Verification items for this drawing (mm, ordinates from the low corner). A direction names the side the tool comes from. Coordinates: 2 decimals unless noted, no trailing zeros. Order: outer loops, then holes, each group sorted by start corner. A loop starts at its lowest first (then second) coordinate and runs counter-clockwise, first axis right, second up. Notation, with made-up numbers: M 63.5,-25 L 81.5,-25 A26 ccw 81.5,0 Z; hole C -16.75,74 d4. An arc over 180 degrees is marked long. Answer as a JSON object with one key per item and string values. Group by question number.
(1) Cross-section at A-A (y = 108). Enter the section's corners in (x, z).
(2) Gauge pin test, flat ends, axial feed: pin 1 Ø5 at (x, y) = (250.83, 7.17) entering from -Z; pin 2 Ø7 at (x, y) = (250.83, 140.83) entering from +Z. Record the tip position at first contact, or that the pin passes through.
(3) Cross-section at B-B (x = 163). Enter the section's corners in (y, z).
(4) Cross-section at C-C (z = 27.5). Enter the section's corners in (x, y), plus the area to 3 significant figures.
(5) Access from +Z, -Z, +X, -X, +Y, -Y to the whole of each face (thin tool, end or side, straight path). Record for the marked faces 1 and 2.
(6) Material ranges on line 1 (Y direction, x = 87, z = 37); line 2 (X direction, y = 78, z = 31.5); line 3 (X direction, y = 140.5, z = 22), recorded low to high.
(7) Mould release check, pull along Y, two halves, no side actions. Record for the marked faces 3, 4, 5 and 6: released by +Y, released by -Y, zero draft, split by the parting line, or undercut.
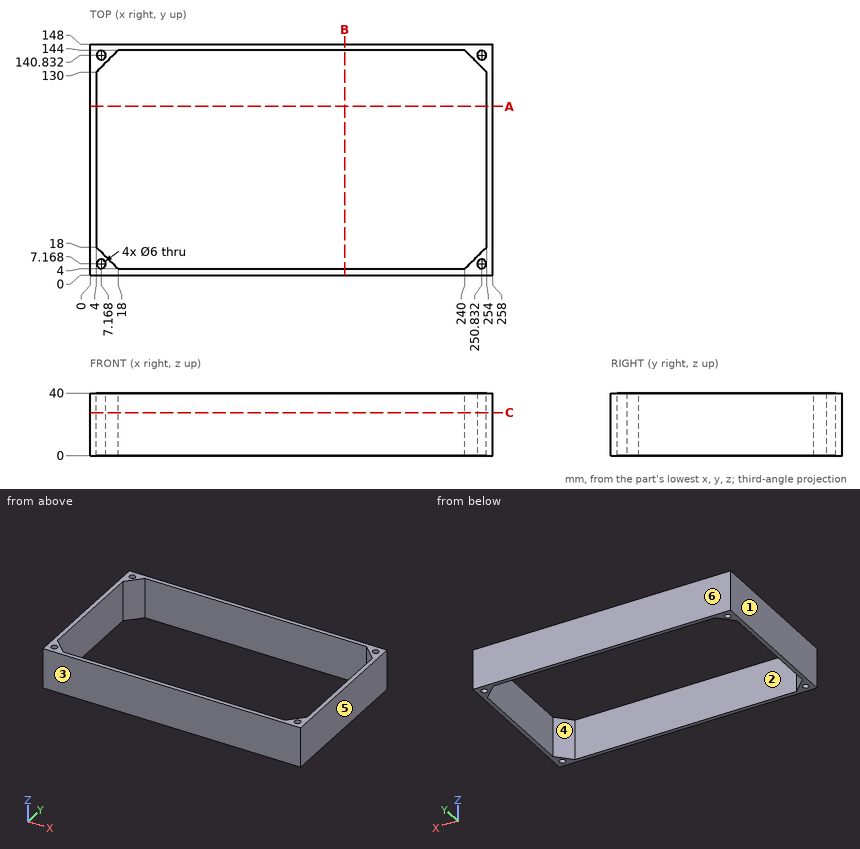
Taken from the geometry:
{
 "1": {"outline": "M 0,0 L 4,0 L 4,40 L 0,40 Z; M 254,0 L 258,0 L 258,40 L 254,40 Z"},
 "2": {"pin 1": "passes through", "pin 2": "stops at z = 40"},
 "3": {"outline": "M 0,0 L 4,0 L 4,40 L 0,40 Z; M 144,0 L 148,0 L 148,40 L 144,40 Z"},
 "4": {"outline": "M 0,0 L 258,0 L 258,148 L 0,148 Z; hole M 4,18 L 18,4 L 240,4 L 254,18 L 254,130 L 240,144 L 18,144 L 4,130 Z; hole C 7.17,7.17 d6; hole C 7.17,140.83 d6; hole C 250.83,7.17 d6; hole C 250.83,140.83 d6", "area": "3,460 mm²"},
 "5": {"face 1": "+Z, -Z, -X, +Y, -Y", "face 2": "+Z, -Z"},
 "6": {"line 1": "y = 0 to 4, 144 to 148", "line 2": "x = 0 to 4, 254 to 258", "line 3": "x = 0 to 4.19, 10.15 to 14.5, 243.5 to 247.85, 253.81 to 258"},
 "7": {"face 3": "released by -Y", "face 4": "undercut", "face 5": "zero draft", "face 6": "released by +Y"}
}
